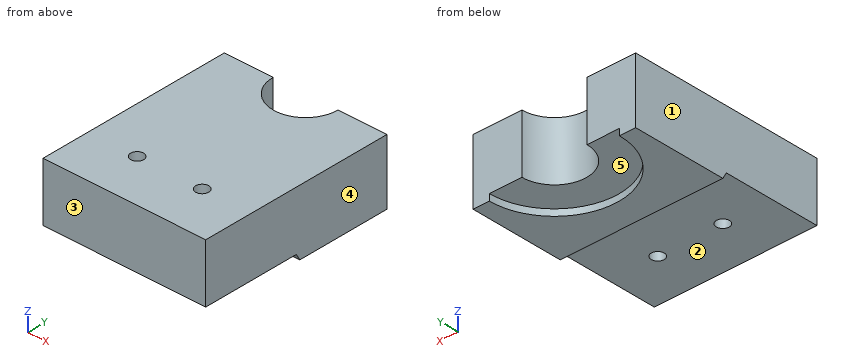
```python
from build123d import *

# Parameters (mm, degrees)
SKETCH1_W           = 25
SKETCH1_H           = 30
BOSS_EXTRUDE1_DEPTH = 10
CUT_EXTRUDE1_DEPTH  = 41.311288741
CUT_EXTRUDE2_DEPTH  = 1
CUT_EXTRUDE3_DEPTH  = 41.074929819
SKETCH5_R           = 1
CUT_EXTRUDE5_DEPTH  = 41.074929819


with BuildPart() as part:
    # Sketch1 → Boss-Extrude1 (new body)
    with BuildSketch(Plane.XY):
        with Locations((12.5, 15)):
            Rectangle(SKETCH1_W, SKETCH1_H)
    extrude(amount=BOSS_EXTRUDE1_DEPTH)

    # Sketch2 → Cut-Extrude1 (cut, through all)
    with BuildSketch(Plane(origin=(25, 0, 0), x_dir=(0, 0, -1), z_dir=(1, 0, 0))):
        Polygon((0, 15.577350269), (-1, 15), (-1, 0), (0, 0), align=None)
    extrude(amount=-CUT_EXTRUDE1_DEPTH, mode=Mode.SUBTRACT)

    # Sketch3 → Cut-Extrude2 (cut)
    with BuildSketch(Plane(origin=(0, 0, 0), x_dir=(-1, 0, 0), z_dir=(0, 0, -1))):
        with BuildLine():
            Line((-22.5, 30), (-2.5, 30))
            ThreePointArc((-2.5, 30), (-12.5, 20), (-22.5, 30))
        make_face()
    extrude(amount=-CUT_EXTRUDE2_DEPTH, mode=Mode.SUBTRACT)

    # Sketch4 → Cut-Extrude3 (cut, through all)
    with BuildSketch(Plane(origin=(0, 0, 1), x_dir=(-1, 0, 0), z_dir=(0, 0, -1))):
        with BuildLine():
            Line((-7.5, 30), (-17.5, 30))
            ThreePointArc((-17.5, 30), (-12.5, 25), (-7.5, 30))
        make_face()
    extrude(amount=-CUT_EXTRUDE3_DEPTH, mode=Mode.SUBTRACT)

    # Sketch5 → Cut-Extrude5 (cut, through all)
    with BuildSketch(Plane(origin=(0, 0, 1), x_dir=(-1, 0, 0), z_dir=(0, 0, -1))):
        with Locations(Location((-17.5, 7.5, 0), (0, 0, 90))):
            Circle(SKETCH5_R)
        with Locations(Location((-7.5, 7.5, 0), (0, 0, 270))):
            Circle(SKETCH5_R)
    extrude(amount=-CUT_EXTRUDE5_DEPTH, mode=Mode.SUBTRACT)


solid = part.part
```
Could you check a few things on this model? Use its own coordinates, in mm. Face numbers are marked on the shaded views. A direction names the side the tool comes from. Round coordinates to 2 decimals unless told otherwise and drop trailing zeros. Loops run counter-clockwise (first coordinate to the right, second up) from the corner with the lowest first, then second, coordinate; pieces in that order, holes last. Notation, with made-up numbers: (84.25, 85.5) - (93.25, 85.5) arc R22 ccw to (93.25, 111.5) - close; hole circle Ø5 at (3, 51). An arc over 180 degrees is marked (long way). Answer in a Markdown table with one row per item. Add a question column.
(1) If we mould it in two halves opening along X, with no side actions, what happens to the marked faces 3, 4 and 5? For each: pulls with the +X half, pulls with the -X half, needs draft (parallel to the pull), parting line crosses it, or undercut.
(2) If we section it at D-D (y = 26.75): Please give me the cut outline in (x, z).
(3) I need wall thicknesses on line 1 along X through (y, z) = (7.5, 4); line 2 along Y through (x, z) = (12.5, 2.5); line 3 along Z through (x, y) = (10, 3). Which ranges of each line are inside material? Lowest first, please.
(4) For the marked faces 1 and 2, which set-ups out of +Z, -Z, +X, -X, +Y, -Y let a thin tool reach every point of the face, with its end or its side?
(5) I'm going to push flat-ended pins straight in: pin 1 (7.5 mm diameter, centred on x = 13.5, y = 10.5, fed in from -Z); pin 2 (1.6 mm diameter, centred on x = 17.5, y = 7.5, fed in from +Z). Where does each tip first touch, or does it pass through?
(6) If we section it at C-C (x = 12.5): Please give me the cut outline in (y, z), plus the area to 3 significant figures.
(7) If we section it at A-A (z = 4.5): Please give me the cut outline in (x, y), plus the area to 3 significant figures.
(8) If we section it at B-B (y = 7.5): Please give me the cut outline in (x, z), plus the area to 3 significant figures.
Model answer:
| question | item | result |
|---|---|---|
| 1 | face 3 | needs draft |
| 1 | face 4 | pulls with the +X half |
| 1 | face 5 | undercut |
| 2 | outline | (0, 0) - (3.04, 0) - (3.04, 1) - (8.7, 1) - (8.7, 10) - (0, 10) - close; (16.3, 1) - (21.96, 1) - (21.96, 0) - (25, 0) - (25, 10) - (16.3, 10) - close |
| 3 | line 1 | x = 0 to 6.5, 8.5 to 16.5, 18.5 to 25 |
| 3 | line 2 | y = 0 to 25 |
| 3 | line 3 | z = 1 to 10 |
| 4 | face 1 | +Z, -Z, -X, +Y, -Y |
| 4 | face 2 | -Z, +X, -X, -Y |
| 5 | pin 1 | stops at z = 1 |
| 5 | pin 2 | passes through |
| 6 | outline | (0, 1) - (15, 1) - (15.58, 0) - (20, 0) - (20, 1) - (25, 1) - (25, 10) - (0, 10) - close |
| 6 | area | 230 mm² |
| 7 | outline | (0, 0) - (25, 0) - (25, 30) - (17.5, 30) arc R5 cw to (7.5, 30) - (0, 30) - close; hole circle Ø2 at (7.5, 7.5); hole circle Ø2 at (17.5, 7.5) |
| 7 | area | 704 mm² |
| 8 | outline | (0, 1) - (6.5, 1) - (6.5, 10) - (0, 10) - close; (8.5, 1) - (16.5, 1) - (16.5, 10) - (8.5, 10) - close; (18.5, 1) - (25, 1) - (25, 10) - (18.5, 10) - close |
| 8 | area | 189 mm² |
